The model under review builds one solid part; all positions refer to its coordinate system, in mm. Face numbers are marked on the shaded views. A direction names the side the tool comes from. Coordinates: 2 decimals unless noted, no trailing zeros. Write each loop counter-clockwise with the first axis right and the second up, starting at its lowest first coordinate (ties: lowest second). Pieces come first, ordered by that corner, then holes.
```python
from build123d import *

# Parameters (mm, degrees)
SKETCH2_W           = 33
SKETCH2_H           = 37.5
BOSS_EXTRUDE1_DEPTH = 5
SKETCH3_W           = 33
SKETCH3_H           = 5
BOSS_EXTRUDE2_DEPTH = 20
SKETCH6_R           = 2.65
CUT_EXTRUDE2_DEPTH  = 10
SKETCH7_R           = 2.65
CUT_EXTRUDE3_DEPTH  = 10
SKETCH8_W           = 4.5
SKETCH8_H           = 12.5
BOSS_EXTRUDE3_DEPTH = 25
SKETCH9_R           = 2.2
CUT_EXTRUDE4_DEPTH  = 10


with BuildPart() as part:
    # Sketch2 → Boss-Extrude1 (new body)
    with BuildSketch(Plane.XY):
        with Locations((16.5, 18.75)):
            Rectangle(SKETCH2_W, SKETCH2_H)
    extrude(amount=BOSS_EXTRUDE1_DEPTH)

    # Sketch3 → Boss-Extrude2 (add)
    with BuildSketch(Plane.XY):
        with Locations((16.5, 2.5)):
            Rectangle(SKETCH3_W, SKETCH3_H)
    extrude(amount=-BOSS_EXTRUDE2_DEPTH)

    # Sketch6 → Cut-Extrude2 (cut)
    with BuildSketch(Plane.XZ):
        with Locations(Location((16.5, -10, 0), (0, 0, 270))):
            Circle(SKETCH6_R)
    extrude(amount=-CUT_EXTRUDE2_DEPTH, mode=Mode.SUBTRACT)

    # Sketch7 → Cut-Extrude3 (cut)
    with BuildSketch(Plane(origin=(0, 0, 0), x_dir=(-1, 0, 0), z_dir=(0, 0, -1))):
        with Locations((-16.5, 15)):
            Circle(SKETCH7_R)
    extrude(amount=-CUT_EXTRUDE3_DEPTH, mode=Mode.SUBTRACT)

    # Sketch8 → Boss-Extrude3 (add)
    with BuildSketch(Plane(origin=(0, 0, 0), x_dir=(-1, 0, 0), z_dir=(0, 0, -1))):
        with Locations((-30.75, 31.25)):
            Rectangle(SKETCH8_W, SKETCH8_H)
        with Locations((-2.25, 31.25)):
            Rectangle(SKETCH8_W, SKETCH8_H)
    extrude(amount=BOSS_EXTRUDE3_DEPTH)

    # Sketch9 → Cut-Extrude4 (cut)
    with BuildSketch(Plane.XY.offset(5)):
        with Locations((16.5, 31.25)):
            Circle(SKETCH9_R)
    extrude(amount=-CUT_EXTRUDE4_DEPTH, mode=Mode.SUBTRACT)


solid = part.part
```
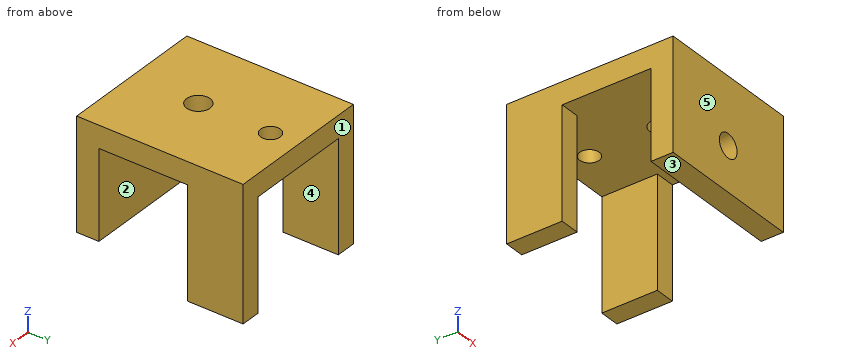
Item 1: Take a section at C-C, the plane x = 16.5. Write out the cut boundary in (y, z), plus the area to 4 significant figures.
Solved:
outline: (0, -20) - (5, -20) - (5, -12.65) - (0, -12.65) - close; (0, -7.35) - (5, -7.35) - (5, 0) - (12.35, 0) - (12.35, 5) - (0, 5) - close; (17.65, 0) - (29.05, 0) - (29.05, 5) - (17.65, 5) - close; (33.45, 0) - (37.5, 0) - (37.5, 5) - (33.45, 5) - close
area: 212.5 mm2
Item 2: To check wall thickness, follow line 1 along Y through (x, z) = (16.5, 2.2); line 2 along X through (y, z) = (1.75, -10); line 3 along X through (y, z) = (27, -15.25). State the ranges of each line that lie inside material, in increasing order.
Solved:
line 1: y = 0 to 12.35, 17.65 to 29.05, 33.45 to 37.5
line 2: x = 0 to 13.85, 19.15 to 33
line 3: x = 0 to 4.5, 28.5 to 33
Item 3: Mouldability with a two-part tool opening along Y and no side actions: class the marked faces 1, 2 and 3 as pulls with the +Y half, pulls with the -Y half, needs draft (parallel to the pull), parting line crosses it, or undercut.
Solved:
face 1: pulls with the +Y half
face 2: undercut
face 3: needs draft
Item 4: Take a section at D-D, the plane z = -10. Write out the cut boundary in (x, y), plus the area to 3 significant figures.
Solved:
outline: (0, 0) - (13.85, 0) - (13.85, 5) - (0, 5) - close; (0, 25) - (4.5, 25) - (4.5, 37.5) - (0, 37.5) - close; (19.15, 0) - (33, 0) - (33, 5) - (19.15, 5) - close; (28.5, 25) - (33, 25) - (33, 37.5) - (28.5, 37.5) - close
area: 251 mm2
Item 5: Take a section at B-B, the plane y = 31.25. Write out the cut boundary in (x, z), plus the area to 3 significant figures.
Solved:
outline: (0, -25) - (4.5, -25) - (4.5, 0) - (14.3, 0) - (14.3, 5) - (0, 5) - close; (18.7, 0) - (28.5, 0) - (28.5, -25) - (33, -25) - (33, 5) - (18.7, 5) - close
area: 368 mm2
Item 6: Take a section at A-A, the plane z = -17.25. Write out the cut boundary in (x, y), plus the area to 4 significant figures.
Solved:
outline: (0, 0) - (33, 0) - (33, 5) - (0, 5) - close; (0, 25) - (4.5, 25) - (4.5, 37.5) - (0, 37.5) - close; (28.5, 25) - (33, 25) - (33, 37.5) - (28.5, 37.5) - close
area: 277.5 mm2
Item 7: Machinability: for the marked faces 4 and 5, which of the approach directions +Z, -Z, +X, -X, +Y, -Y give a long, thin tool a straight path to every point of the face, cutting with its end or side? Answer none if there is none.
Solved:
face 4: -Z, +Y
face 5: +Z, -Z, +X, -X, -Y
Item 8: For pin 1 (7 mm diameter, centred on x = 16.5, y = 15, fed in from +Z); pin 2 (2 mm diameter, centred on x = 27.5, y = 15.5, fed in from -Z); pin 3 (10 mm diameter, centred on x = 15.5, z = -8, fed in from +Y); pin 4 (4 mm diameter, centred on x = 21, y = 1.5, fed in from -Z), all flat-tipped, find the tip position at first contact; note any pin that passes through.
Solved:
pin 1: stops at z = 5
pin 2: stops at z = 0
pin 3: stops at y = 5
pin 4: stops at z = -20
